Could you check a few things on this model? Use its own coordinates, in mm. Face numbers are marked on the shaded views. A direction names the side the tool comes from. Give positions to 0.01 mm unless a question says otherwise; leave off trailing zeros. Order: outer loops, then holes, each group sorted by start corner. A loop starts at its lowest first (then second) coordinate and runs counter-clockwise, first axis right, second up. Notation, with made-up numbers: (5.5, 27) -> (13.5, 27) arc R18 cw to (13.5, 33) -> close; hole circle Ø11 at (66, 61). An arc over 180 degrees is marked (long way). Use one line per item in the form item = value. Start each with the question number.
Autodesk Inventor part; units mm, degrees
ref_plane "YZ Plane" through (0, 0, 0) normal (1, 0, 0) x (0, 1, 0)
ref_plane "XZ Plane" through (0, 0, 0) normal (0, 1, 0) x (-1, 0, 0)
ref_plane "XY Plane" through (0, 0, 0) normal (0, 0, 1) x (1, 0, 0)
sketch "Sketch1" plane through (0, 0, 0) normal (0, 0, 1) x (1, 0, 0)
  line L0 (-8, 16) -> (8, 16)
  line L1 (8, 16) -> (8, -16)
  line L2 (8, -16) -> (-8, -16)
  line L3 (-8, -16) -> (-8, 16)
  point P0 (0, 0)
  dimension "d0" = 16
  dimension "d1" = 32
  dimension "d2" = 8
  dimension "d3" = 16
extrude "Extrusion1" add sketch "Sketch1" along normal blind 9.6
shell "Shell1" thickness 1.5 removed faces 1 at (-2.6667, -5.3333, 0)
sketch "Sketch2" plane through (0, 0, 9.6) normal (0, 0, 1) x (1, 0, 0)
  circle A0 centre (4, -12) radius 2.5
  line L0 (8, 16) -> (8, -16)
  line L1 (8, -16) -> (-8, -16)
  dimension "d7" = 5
  dimension "d10" = 4
  dimension "d11" = 4
extrude "Extrusion2" add sketch "Sketch2" along normal blind 1.6
sketch "Sketch3" plane through (6.5, -14.5, 8.1) normal (0, 0, -1) x (-1, 0, 0)
  circle A0 centre (2.5, 2.5) radius 2.5
  circle A1 centre (2.5, 2.5) radius 1.2
  point P0 (6.5, 14.5)
  dimension "d18" = 2.4
extrude "Extrusion3" cut sketch "Sketch3" against normal blind 1.6 contours A1
pattern_linear "Rectangular Pattern1" count 4 spacing 8 along (0, 1, 0) count 2 spacing 8 along (-1, 0, 0) of "Extrusion2", "Extrusion3"
sketch "Sketch4" plane through (6.5, -14.5, 8.1) normal (0, 0, -1) x (-1, 0, 0)
  circle A0 centre (2.5, 10.5) radius 1.2
  circle A1 centre (2.5, 2.5) radius 1.2
  line L0 (0, 29) -> (0, 0)
  line L1 (0, 0) -> (13, 0)
  circle A2 centre (6.5, 6.5) radius 3.15
  circle A3 centre (6.5, 6.5) radius 2.5
  point P0 (6.5, 14.5)
  dimension "d21" = 6.5
  dimension "d22" = 6.5
  dimension "d23" = 10.5
  dimension "d24" = 2.5
  dimension "d25" = 5
  dimension "d26" = 6.3
extrude "Extrusion4" add sketch "Sketch4" along normal up to surface (8.1 mm away) contours A2
pattern_linear "Rectangular Pattern2" count 3 spacing 8 along (0, 1, 0) of "Extrusion4"
equation "\"d0\" = 0.8 * WIDTH"
equation "\"d1\" = 0.8 * LENGTH"
equation "\"d21\" = 0.5 * d23 + 0.5 * d24"
equation "\"d22\" = d21"
equation "\"WIDTH\" = 2"
properties part number "3001" material "Steel"
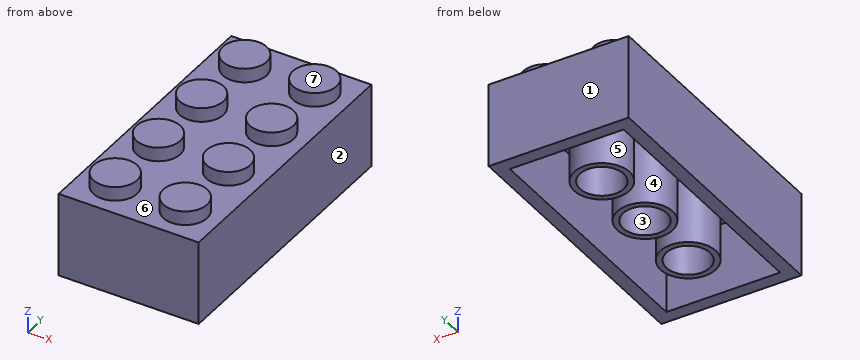
(1) Please list where these lines run through material, in increasing order: probe 1 along Y at (x, z) = (-4, 8.9); probe 2 along X at (y, z) = (-1, 5.75); probe 3 along X at (y, z) = (-13, 3.25).
(2) Imagine slicing it at A-A (z = 1.5). Write out the boundary of the cut face in (x, y), plus the area to 3 significant figures.
(3) We'd pull the mould along Y, two halves only. Please class the marked faces 1, 2, 3 and 4: pulls with the +Y half, pulls with the -Y half, needs draft (parallel to the pull), parting line crosses it, or undercut.
(4) Imagine slicing it at B-B (y = 13.5). Write out the boundary of the cut face in (x, z).
(5) I'm going to push flat-ended pins straight in: pin 1 Ø2.5 at (x, y) = (-3.5, 3.5) entering from -Z; pin 2 Ø2 at (x, y) = (4, 4) entering from -Z; pin 3 Ø5 at (x, y) = (0, 12) entering from +Z. Where does each tip first touch, or does it pass through?
(6) Imagine slicing it at C-C (z = 8.5). Give the number of separate pieces and of enclosed holes in the cut face, plus the area to 3 significant figures.
(7) Which directions (+Z, -Z, +X, -X, +Y, -Y) give clear straight access to the entire face, cutting with the end or side of a thin tool? Please do the marked faces 5, 6 and 7.
Calculated:
q1.probe_1 = -16 to -13.2, -10.8 to -5.2, -2.8 to 2.8, 5.2 to 10.8, 13.2 to 16
q1.probe_2 = -8 to -6.5, -2.99 to -2.29, 2.29 to 2.99, 6.5 to 8
q1.probe_3 = -8 to -6.5, 6.5 to 8
q2.outline = (-8, -16) -> (8, -16) -> (8, 16) -> (-8, 16) -> close; circle Ø6.3 at (0, -8); circle Ø6.3 at (0, 0); circle Ø6.3 at (0, 8); hole (-6.5, -14.5) -> (6.5, -14.5) -> (6.5, 14.5) -> (-6.5, 14.5) -> close; hole circle Ø5 at (0, -8); hole circle Ø5 at (0, 0); hole circle Ø5 at (0, 8)
q2.area = 170 mm2
q3.face_1 = pulls with the +Y half
q3.face_2 = needs draft
q3.face_3 = undercut
q3.face_4 = undercut
q4.outline = (-8, 0) -> (-6.5, 0) -> (-6.5, 8.1) -> (6.5, 8.1) -> (6.5, 0) -> (8, 0) -> (8, 9.6) -> (6, 9.6) -> (6, 11.2) -> (2, 11.2) -> (2, 9.6) -> (-2, 9.6) -> (-2, 11.2) -> (-6, 11.2) -> (-6, 9.6) -> (-8, 9.6) -> close
q5.pin_1 = 8.1
q5.pin_2 = 9.7
q5.pin_3 = 11.2
q6.separate_pieces = 1
q6.enclosed_holes = 8
q6.area = 476 mm2
q7.face_5 = -Z
q7.face_6 = +Z
q7.face_7 = +Z, +X, -X, +Y, -Y
